Work out the finished part from the listing and answer in its coordinate system (mm). A direction names the side the tool comes from. Round coordinates to 2 decimals unless told otherwise and drop trailing zeros. Write each loop counter-clockwise with the first axis right and the second up, starting at its lowest first coordinate (ties: lowest second). Pieces come first, ordered by that corner, then holes.
1. A tool of negligible diameter and unlimited length cuts with its end or side. For faces 1 (the face through (10.17, 0.16, 0.03)), 2 (the face through (95.754, 12.239, 0.028)), from which of +Z, -Z, +X, -X, +Y, -Y can it reach the whole face along a straight path? Write none if from no direction.
2. Find section C-C (y = 16.5). Write down the section's boundary in (x, z), and give its area (3 significant figures).
3. Find section B-B (x = 102). Write down the section's boundary in (y, z), and give its area (3 significant figures).
4. Find section A-A (z = 0.65). Count the separate pieces of the cut face and the enclosed holes in it, and give its area (3 significant figures).
5. Straight lines are drawn through the part: probe 1 along X at (y, z) = (3.5, 0.85); probe 2 along Y at (x, z) = (94.5, 0.75); probe 3 along X at (y, z) = (10, -1.05). For each, find the intervals that lie inside material, in ascending order.
6. Flat-ended cylindrical pins translate along their axes: pin 1 Ø1 at (y, z) = (8.5, 1) entering from -X; pin 2 Ø4 at (x, y) = (121.12, -2.62) entering from -Z; pin 3 Ø1.5 at (x, z) = (101, -1.5) entering from +Y. Find the tip coordinate at first contact, or state that the pin passes through.
7. Determine the mould class of faces 3 (the face through (124.826, 11.612, -0.028)), 4 (the face through (59, 7, -2)), 5 (the face through (67.43, -1.438, 0.028)), 6 (the face through (-5.716, 12.07, 0.028)) for opening direction X: pulls with the +X half, pulls with the -X half, needs draft (parallel to the pull), parting line crosses it, or undercut.
```python
from build123d import *

# Parameters (mm, degrees)
SKETCH_1_R          = 6
EXTRUDE_1_DEPTH     = 2
SKETCH_2_R          = 1.55
SKETCH_2_R_2        = 0.6
CUT_EXTRUDE_1_DEPTH = 5
FILLET_1_R          = 3.5
CUT_EXTRUDE_2_DEPTH = 5
SKETCH_4_R          = 1.55
CUT_EXTRUDE_3_DEPTH = 5
FILLET_2_R          = 3.5


with BuildPart() as part:
    # 草图1 → 凸台-拉伸1 (new body, symmetric)
    with BuildSketch(Plane.XY):
        with BuildLine():
            Line((-8.927079897, 3.249191362), (-1.4961968, 23.665374879))
            Line((-1.4961968, 23.665374879), (160.827979556, 9.463849632))
            ThreePointArc((160.827979556, 9.463849632), (169.463849632, -0.827979556), (159.172020444, -9.463849632))
            Line((159.172020444, -9.463849632), (11.371578553, 3.467013498))
            Line((11.371578553, 3.467013498), (8.927079897, -3.249191362))
            ThreePointArc((8.927079897, -3.249191362), (-3.249191362, -8.927079897), (-8.927079897, 3.249191362))
        make_face()
        Circle(SKETCH_1_R, mode=Mode.SUBTRACT)
        with Locations((160, 0)):
            Circle(SKETCH_1_R, mode=Mode.SUBTRACT)
    extrude(amount=EXTRUDE_1_DEPTH, both=True)

    # 草图2 → 切除-拉伸1 (cut, through all)
    with BuildSketch(Plane.XY.offset(2)):
        with Locations((0.874182871, 19.944624098)):
            Circle(SKETCH_2_R)
        with Locations((16.220555377, 6.556152427)):
            Circle(SKETCH_2_R)
        with Locations((11.935394126, 3.261801412)):
            Circle(SKETCH_2_R_2)
    extrude(amount=-CUT_EXTRUDE_1_DEPTH, mode=Mode.SUBTRACT)

    # 圆角1
    fillet_1_edges = [part.edges().sort_by_distance(p)[0] for p in [
        (-1.4961968, 23.665374879, 0),
    ]]
    fillet(fillet_1_edges, radius=FILLET_1_R)

    # 草图3 → 切除-拉伸2 (cut, through all)
    with BuildSketch(Plane.XY.offset(2)):
        with BuildLine():
            Line((125.961165123, 12.514300628), (124.305206011, -6.413398636))
            Line((124.305206011, -6.413398636), (159.172020444, -9.463849632))
            ThreePointArc((159.172020444, -9.463849632), (169.463849632, -0.827979556), (160.827979556, 9.463849632))
            Line((160.827979556, 9.463849632), (125.961165123, 12.514300628))
        make_face()
    extrude(amount=-CUT_EXTRUDE_2_DEPTH, mode=Mode.SUBTRACT)

    # 草图4 → 切除-拉伸3 (cut, through all)
    with BuildSketch(Plane.XY.offset(2)):
        with Locations((122.16943858, 9.332664284)):
            Circle(SKETCH_4_R)
        with Locations((121.123569667, -2.621672093)):
            Circle(SKETCH_4_R)
        with Locations((94.275987033, 11.773025081)):
            Circle(SKETCH_4_R)
        with Locations((93.23011812, -0.181311296)):
            Circle(SKETCH_4_R)
        with Locations((108.222712807, 10.552844683)):
            Circle(SKETCH_4_R)
        with Locations((107.176843894, -1.401491694)):
            Circle(SKETCH_4_R)
    extrude(amount=-CUT_EXTRUDE_3_DEPTH, mode=Mode.SUBTRACT)

    # 圆角2
    fillet_2_edges = [part.edges().sort_by_distance(p)[0] for p in [
        (125.961165123, 12.514300628, 0),
        (124.305206011, -6.413398636, 0),
    ]]
    fillet(fillet_2_edges, radius=FILLET_2_R)


solid = part.part
```
Worked answers:
1. face 1: +Z, -Z, -Y
1. face 2: +Z, -Z
2. outline: (-4.1, -2) - (80.4, -2) - (80.4, 2) - (-4.1, 2) - close
2. area: 338 mm2
3. outline: (-4.46, -2) - (14.61, -2) - (14.61, 2) - (-4.46, 2) - close
3. area: 76.3 mm2
4. separate pieces: 1
4. enclosed holes: 9
4. area: 2,530 mm2
5. probe 1: x = -8.84 to -4.87, 4.87 to 11.38, 12.49 to 125.17
5. probe 2: y = -3.81 to -1.07, 0.71 to 10.24, 13.31 to 15.27
5. probe 3: x = -6.47 to 106.77, 109.67 to 120.77, 123.57 to 125.61
6. pin 1: stops at x = -7.2
6. pin 2: stops at z = -2
6. pin 3: stops at y = 14.76
7. face 3: pulls with the +X half
7. face 4: needs draft
7. face 5: undercut
7. face 6: pulls with the -X half
